from build123d import *

# Parameters (mm, degrees)
CROQUIS1_R              = 100
SALIENTE_EXTRUIR1_DEPTH = 3
CROQUIS3_R              = 120
CORTAR_EXTRUIR1_DEPTH   = 3
CORTAR_EXTRUIR6_DEPTH   = 10
CROQUIS12_R             = 1.5
CORTAR_EXTRUIR7_DEPTH   = 142.453172464
CROQUIS9_R              = 1.5
CROQUIS9_W              = 9
CROQUIS9_H              = 10
CROQUIS9_W_2            = 10
CROQUIS9_H_2            = 9
CORTAR_EXTRUIR5_DEPTH   = 10
CROQUIS13_R             = 2
CROQUIS13_W             = 45
CROQUIS13_H             = 38
CORTAR_EXTRUIR8_DEPTH   = 142.453172464
REDONDEO2_R             = 3
REDONDEO3_R             = 3
CROQUIS14_R             = 1.5
CORTAR_EXTRUIR9_DEPTH   = 142.453172607


with BuildPart() as part:
    # Croquis1 → Saliente-Extruir1 (new body)
    with BuildSketch(Plane.XY):
        Circle(CROQUIS1_R)
    extrude(amount=SALIENTE_EXTRUIR1_DEPTH)

    # Croquis3 → Cortar-Extruir1 (cut)
    with BuildSketch(Plane.XY.offset(3)):
        with Locations((190, 0)):
            Circle(CROQUIS3_R)
    extrude(amount=-CORTAR_EXTRUIR1_DEPTH, mode=Mode.SUBTRACT)

    # Croquis5 → Cortar-Extruir6 (cut)
    with BuildSketch(Plane.XY.offset(3)):
        Polygon((-58.336309448, -83.085046789), (-83.085046789, -58.336309448), (-65.40737726, -40.658639918), (-40.658639918, -65.40737726), align=None)
        Polygon((-83.085046789, 58.336309448), (-58.336309448, 83.085046789), (-40.658639918, 65.40737726), (-65.40737726, 40.658639918), align=None)
        Polygon((58.336309448, -83.085046789), (83.085046789, -58.336309448), (65.40737726, -40.658639918), (40.658639918, -65.40737726), align=None)
        Polygon((58.336309448, 83.085046789), (83.085046789, 58.336309448), (65.40737726, 40.658639918), (40.658639918, 65.40737726), align=None)
    extrude(amount=-CORTAR_EXTRUIR6_DEPTH, mode=Mode.SUBTRACT)

    # Croquis12 → Cortar-Extruir7 (cut, through all)
    with BuildSketch(Plane.XY.offset(3)):
        with Locations((-63.604254904, -36.804908024)):
            Circle(CROQUIS12_R)
        with Locations((-36.804907897, -63.604255031)):
            Circle(CROQUIS12_R)
        with Locations((-47.666068056, -20.866721176)):
            Circle(CROQUIS12_R)
        with Locations((-20.866721049, -47.666068183)):
            Circle(CROQUIS12_R)
        with Locations(Location((47.666068183, 20.866721049, 0), (0, 0, 180))):
            Circle(CROQUIS12_R)
        with Locations(Location((20.866721176, 47.666068056, 0), (0, 0, 180))):
            Circle(CROQUIS12_R)
        with Locations(Location((63.604255031, 36.804907897, 0), (0, 0, 180))):
            Circle(CROQUIS12_R)
        with Locations(Location((36.804908024, 63.604254904, 0), (0, 0, 180))):
            Circle(CROQUIS12_R)
        with Locations((20.866721325, -47.666067908)):
            Circle(CROQUIS12_R)
        with Locations((47.666068332, -20.866720901)):
            Circle(CROQUIS12_R)
        with Locations((63.60425518, -36.804907749)):
            Circle(CROQUIS12_R)
        with Locations((36.804908173, -63.604254756)):
            Circle(CROQUIS12_R)
        with Locations(Location((-63.604254756, 36.804908173, 0), (0, 0, 180))):
            Circle(CROQUIS12_R)
        with Locations(Location((-36.804907749, 63.60425518, 0), (0, 0, 180))):
            Circle(CROQUIS12_R)
        with Locations(Location((-20.866720901, 47.666068332, 0), (0, 0, 180))):
            Circle(CROQUIS12_R)
        with Locations(Location((-47.666067908, 20.866721325, 0), (0, 0, 180))):
            Circle(CROQUIS12_R)
    extrude(amount=-CORTAR_EXTRUIR7_DEPTH, mode=Mode.SUBTRACT)

    # Croquis9 → Cortar-Extruir5 (cut)
    with BuildSketch(Plane.XY.offset(3)):
        with Locations((52, -4)):
            Circle(CROQUIS9_R)
        with Locations((16, 4)):
            Circle(CROQUIS9_R)
        with Locations((52, 4)):
            Circle(CROQUIS9_R)
        with Locations((16, -4)):
            Circle(CROQUIS9_R)
        with Locations((-85, 4)):
            Circle(CROQUIS9_R)
        with Locations((-85, -4)):
            Circle(CROQUIS9_R)
        with Locations((-49, 4)):
            Circle(CROQUIS9_R)
        with Locations((-49, -4)):
            Circle(CROQUIS9_R)
        with Locations((-4, 85)):
            Circle(CROQUIS9_R)
        with Locations((4, 85)):
            Circle(CROQUIS9_R)
        with Locations((-4, 49)):
            Circle(CROQUIS9_R)
        with Locations((4, 49)):
            Circle(CROQUIS9_R)
        with Locations((-4, -49)):
            Circle(CROQUIS9_R)
        with Locations((4, -49)):
            Circle(CROQUIS9_R)
        with Locations((4, -85)):
            Circle(CROQUIS9_R)
        with Locations((-4, -85)):
            Circle(CROQUIS9_R)
        with Locations((24.5, 0)):
            Rectangle(CROQUIS9_W, CROQUIS9_H)
        with Locations((0, -57.5)):
            Rectangle(CROQUIS9_W_2, CROQUIS9_H_2)
        with Locations((-57.5, 0)):
            Rectangle(CROQUIS9_W, CROQUIS9_H)
        with Locations((0, 57.5)):
            Rectangle(CROQUIS9_W_2, CROQUIS9_H_2)
    extrude(amount=-CORTAR_EXTRUIR5_DEPTH, mode=Mode.SUBTRACT)

    # Croquis13 → Cortar-Extruir8 (cut, through all)
    with BuildSketch(Plane.XY.offset(3)):
        with Locations((-70.710287698, 30)):
            Circle(CROQUIS13_R)
        with Locations((-70.709712289, -30)):
            Circle(CROQUIS13_R)
        with Locations((0, -92)):
            Circle(CROQUIS13_R)
        with Locations((0, 92)):
            Circle(CROQUIS13_R)
        with Locations((60, -20)):
            Circle(CROQUIS13_R)
        with Locations((60, 20)):
            Circle(CROQUIS13_R)
        with Locations((-14.5, 1)):
            Rectangle(CROQUIS13_W, CROQUIS13_H)
    extrude(amount=-CORTAR_EXTRUIR8_DEPTH, mode=Mode.SUBTRACT)

    # Redondeo2
    # the kernel refuses this fillet: 3 mm, written as the material it adds along each edge
    with BuildSketch(Plane(origin=(-37, -18, 3), x_dir=(0, 1, 0), z_dir=(0, 0, -1)), Plane(origin=(8, 20, 3), x_dir=(0, -1, 0), z_dir=(0, 0, -1)), Plane(origin=(8, -18, 3), x_dir=(-1, 0, 0), z_dir=(0, 0, -1)), Plane(origin=(40.658639918, -65.40737726, 3), x_dir=(0.7071067811865925, 0.7071067811865025, 0), z_dir=(0, 0, -1)), Plane(origin=(65.40737726, -40.658639918, 3), x_dir=(0.7071067811865014, -0.7071067811865938, 0), z_dir=(0, 0, -1)), Plane(origin=(-40.658639918, -65.40737726, 3), x_dir=(-0.7071067811865688, -0.7071067811865261, 0), z_dir=(0, 0, -1)), Plane(origin=(-65.40737726, -40.658639918, 3), x_dir=(0.7071067811865263, -0.7071067811865689, 0), z_dir=(0, 0, -1))) as redondeo2_piece_1:
        with BuildLine():
            CenterArc((REDONDEO2_R, REDONDEO2_R), REDONDEO2_R, 180, 90)
            Line((0, REDONDEO2_R), (0, 0))
            Line((0, 0), (REDONDEO2_R, 0))
        make_face()
    extrude(amount=3)
    with BuildSketch(Plane(origin=(-37, 20, 3), x_dir=(0, -1, 0), z_dir=(0, 0, -1)), Plane(origin=(-40.658639918, 65.40737726, 3), x_dir=(-0.7071067811865013, 0.7071067811865936, 0), z_dir=(0, 0, -1)), Plane(origin=(-65.40737726, 40.658639918, 3), x_dir=(0.707106781186595, 0.7071067811865002, 0), z_dir=(0, 0, -1)), Plane(origin=(40.658639918, 65.40737726, 3), x_dir=(0.707106781186525, -0.70710678118657, 0), z_dir=(0, 0, -1)), Plane(origin=(65.40737726, 40.658639918, 3), x_dir=(0.7071067811865688, 0.7071067811865261, 0), z_dir=(0, 0, -1))) as redondeo2_piece_2:
        with BuildLine():
            CenterArc((REDONDEO2_R, -REDONDEO2_R), REDONDEO2_R, 90, 90)
            Line((0, -REDONDEO2_R), (0, 0))
            Line((0, 0), (REDONDEO2_R, 0))
        make_face()
    extrude(amount=3)
    # the kernel refuses this fillet: 3 mm, written as the material it takes off along each edge
    with BuildSketch(Plane(origin=(-81.993870249, 57.245132907, 12.259512252), x_dir=(0.7071067811864988, -0.7071067811865962, 0), z_dir=(0, 0, -1)), Plane(origin=(57.245132907, 81.993870249, 12.259512252), x_dir=(-0.707106781186567, -0.707106781186528, 0), z_dir=(0, 0, -1))) as redondeo2_2_piece_1:
        with BuildLine():
            CenterArc((3.647824779, 3), REDONDEO2_R, 167.799096685, 102.200903315)
            ThreePointArc((0.715587092, 3.634020619), (0.340967474, 1.820323587), (0, 0))
            Line((0, 0), (3.647824779, 0))
        make_face()
    extrude(amount=21.519024503, mode=Mode.SUBTRACT)
    with BuildSketch(Plane(origin=(-57.245132907, 81.993870249, 12.259512252), x_dir=(0.8303993298839993, 0.5571686934207671, 0), z_dir=(0, 0, -1))) as redondeo2_2_piece_2:
        with BuildLine():
            CenterArc((3.648247827, 2.999485524), REDONDEO2_R, 168.860219289, 102.200903315)
            Line((0.704771551, 3.579095232), (0, 0))
            ThreePointArc((0, 0), (1.85190245, -0.017149184), (3.703804901, 0))
        make_face()
    extrude(amount=21.519024503, mode=Mode.SUBTRACT)
    with BuildSketch(Plane(origin=(57.245132907, -81.993870249, 12.259512252), x_dir=(-0.7071067811864988, 0.7071067811865962, 0), z_dir=(0, 0, -1)), Plane(origin=(-81.993870249, -57.245132907, 12.259512252), x_dir=(0.707106781186568, 0.707106781186527, 0), z_dir=(0, 0, -1))) as redondeo2_2_piece_3:
        with BuildLine():
            CenterArc((3.647824779, -3), REDONDEO2_R, 90, 102.200903315)
            ThreePointArc((0.715587092, -3.634020619), (0.340967474, -1.820323587), (0, 0))
            Line((0, 0), (3.647824779, 0))
        make_face()
    extrude(amount=21.519024503, mode=Mode.SUBTRACT)
    with BuildSketch(Plane(origin=(81.993870249, -57.245132907, 11.583056929), x_dir=(0.5619940188878753, 0.8271412955077593, 0), z_dir=(0, 0, -1))) as redondeo2_2_piece_4:
        with BuildLine():
            CenterArc((3.590487142, -2.809879123), REDONDEO2_R, 110.507494251, 80.298695839)
            Line((0.643686139, -3.372341435), (0, 0))
            ThreePointArc((0, 0), (1.269748729, 0.008061634), (2.539497458, 0))
        make_face()
    extrude(amount=20.166113858, mode=Mode.SUBTRACT)
    with BuildSketch(Plane(origin=(81.993870249, 57.245132907, 11.583056929), x_dir=(0.5619940188878358, -0.827141295507786, 0), z_dir=(0, 0, -1))) as redondeo2_2_piece_5:
        with BuildLine():
            CenterArc((3.590487142, 2.809879123), REDONDEO2_R, 169.19380991, 80.298695839)
            Line((0.643686139, 3.372341435), (0, 0))
            ThreePointArc((0, 0), (1.269748729, -0.008061634), (2.539497458, 0))
        make_face()
    extrude(amount=20.166113858, mode=Mode.SUBTRACT)
    with BuildSketch(Plane(origin=(-57.245132907, -81.993870249, 12.259512252), x_dir=(0.8303993298839483, -0.5571686934208434, 0), z_dir=(0, 0, -1))) as redondeo2_2_piece_6:
        with BuildLine():
            CenterArc((3.648247827, -2.999485524), REDONDEO2_R, 88.938877397, 102.200903315)
            Line((0.704771551, -3.579095232), (0, 0))
            ThreePointArc((0, 0), (1.85190245, 0.017149184), (3.703804901, 0))
        make_face()
    extrude(amount=21.519024503, mode=Mode.SUBTRACT)

    # Redondeo3
    redondeo3_edges = [part.edges().sort_by_distance(p)[0] for p in [
        (83.421052632, -55.14460969, 1.5),
        (83.421052632, 55.14460969, 1.5),
    ]]
    fillet(redondeo3_edges, radius=REDONDEO3_R)

    # Croquis14 → Cortar-Extruir9 (cut, through all)
    with BuildSketch(Plane.XY.offset(3)):
        with Locations((46.390099465, -78.209904618)):
            Circle(CROQUIS14_R)
        with Locations((-46.613889508, -78.433694662)):
            Circle(CROQUIS14_R)
        with Locations((-78.318210918, -46.498405764)):
            Circle(CROQUIS14_R)
        with Locations((-78.455342963, 46.63553781)):
            Circle(CROQUIS14_R)
        with Locations((-46.498405821, 78.318210974)):
            Circle(CROQUIS14_R)
        with Locations((46.63553784, 78.455342993)):
            Circle(CROQUIS14_R)
    extrude(amount=-CORTAR_EXTRUIR9_DEPTH, mode=Mode.SUBTRACT)


solid = part.part
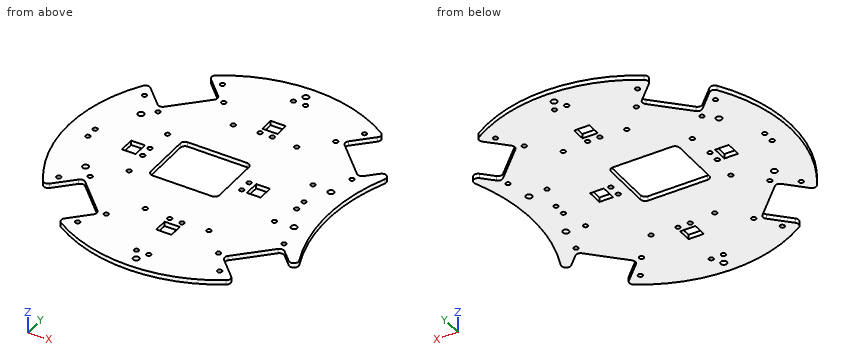
Could you check a few things on this model? Use its own coordinates, in mm. Give positions to 0.01 mm unless a question says otherwise; leave off trailing zeros.
1. Suppose I cut it at A-A (z = 0.95). Give the number of separate pieces and of enclosed holes in the cut face, plus the area to 3 significant figures.
2. I need wall thicknesses on L1, parallel to Y at x = 51, z = 2.85; L2, parallel to X at y = 44, z = 1.6; L3, parallel to Y at x = 38, z = 2.8. Which ranges of each line are inside material? Lowest first, please.
3. Will these pins go through, and if not, where does the flat tip stop? P1, Ø1.5, axis at y = -59.5, z = 2.5, coming from the +X side; P2, Ø0.9, axis at x = 23.5, z = 1.5, coming from the +Y side.
Solved:
1. separate pieces: 1
1. enclosed holes: 49
1. area: 23,300 mm2
2. L1: y = -86.02 to -75.75, -55.07 to -5.12, -2.88 to 2.88, 5.12 to 55.07, 75.75 to 86.02
2. L2: x = -89.8 to -68.75, -62.07 to 62.07, 68.75 to 78.36
2. L3: y = -92.5 to -64.51, -62.7 to 62.7, 64.51 to 92.5
3. P1: stops at x = 47.32
3. P2: stops at y = 97.31
